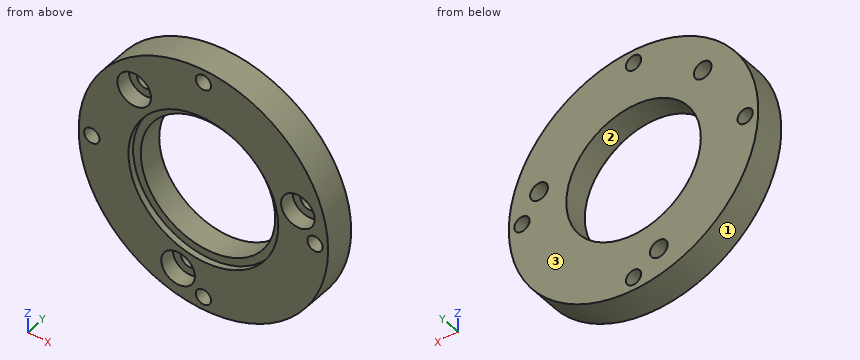
```python
from build123d import *

# Parameters (mm, degrees)
SKETCH_1_R                    = 20.4
SKETCH_1_R_2                  = 11
EXTRUDE_1_DEPTH               = 5
M3X0_51_D                     = 2.5
HOLE_WIZARD_M2_51_D           = 2.9
HOLE_WIZARD_M2_51_CBORE_D     = 5.5
HOLE_WIZARD_M2_51_CBORE_DEPTH = 2.5
SKETCH_9_R                    = 12.25
CUT_EXTRUDE_1_DEPTH           = 1


with BuildPart() as part:
    # Эскиз1 → Бобышка-Вытянуть1 (new body)
    with BuildSketch(Plane(origin=(0, 0, 0), x_dir=(1, 0, 0), z_dir=(0, 1, 0))):
        Circle(SKETCH_1_R)
        Circle(SKETCH_1_R_2, mode=Mode.SUBTRACT)
    extrude(amount=EXTRUDE_1_DEPTH)

    # Отверстие обработанное метчиком M3x0.51 (through all)
    with Locations(Plane(origin=(0, 5, 0), x_dir=(1, 0, 0), z_dir=(0, 1, 0))):
        with Locations((-18.25, 0), (0, 18.25), (18.25, 0), (0, -18.25)):
            Hole(M3X0_51_D / 2)

    # Цековка для винта с внутренним шестигранником M2.51 (through all)
    with Locations(Plane(origin=(0, 0, 0), x_dir=(-1, 0, 0), z_dir=(0, -1, 0))):
        with Locations((11.313708499, -11.313708499), (4.141104722, 15.454813221), (-15.454813221, -4.141104722)):
            CounterBoreHole(HOLE_WIZARD_M2_51_D / 2, HOLE_WIZARD_M2_51_CBORE_D / 2, HOLE_WIZARD_M2_51_CBORE_DEPTH)

    # Эскиз9 → Вырез-Вытянуть1 (cut)
    with BuildSketch(Plane.XZ):
        Circle(SKETCH_9_R)
    extrude(amount=-CUT_EXTRUDE_1_DEPTH, mode=Mode.SUBTRACT)


solid = part.part
```
Source: CAD feature listing. Evaluate the final solid. Frame: model axes, mm. Face numbers are marked on the shaded views. Round coordinates to 2 decimals unless told otherwise and drop trailing zeros. Order: outer loops, then holes, each group sorted by start corner. A loop starts at its lowest first (then second) coordinate and runs counter-clockwise, first axis right, second up. Notation, with made-up numbers: (1.25, 68) -> (49.25, 68) arc R23 ccw to (49.25, 79) -> close; hole circle Ø10 at (4.25, -9). An arc over 180 degrees is marked (long way). One line per item, written item: value. Start each with the question number.
Q1. Pin query (flat end, axial travel): pin 1 (4 mm diameter, centred on x = -18.25, z = 0, fed in from +Y); pin 2 (3.5 mm diameter, centred on x = 15.45, z = 4.14, fed in from -Y). Return the tip coordinate at first contact, or that it passes through.
Q2. Section query C-C (z = 18.25). Return the cut outline in (x, y), plus the area to 3 significant figures.
Q3. Draft query along Z for the marked faces 1, 2 and 3. Return one class per face: pulls with the +Z half, pulls with the -Z half, needs draft (parallel to the pull), parting line crosses it, or undercut.
Q4. Section query B-B (x = -18.25). Return the cut outline in (y, z), plus the area to 3 significant figures.
Q5. Section query D-D (x = 0). Return the cut outline in (y, z).
Q6. Material intervals for probe 1 along Z at (x, y) = (0, 1.1); probe 2 along X at (y, z) = (1.4, 9); probe 3 along X at (y, z) = (2, -17.5), sorted ascending.
Q7. Section query A-A (z = 5). Return the cut outline in (x, y), plus the area to 3 significant figures.
Findings below:
1. pin 1: y = 5
1. pin 2: y = 2.5
2. outline: (-9.12, 0) -> (-1.25, 0) -> (-1.25, 5) -> (-9.12, 5) -> close; (1.25, 0) -> (9.12, 0) -> (9.12, 5) -> (1.25, 5) -> close
2. area: 78.7 mm²
3. face 1: parting line crosses it
3. face 2: undercut
3. face 3: needs draft
4. outline: (0, -9.12) -> (5, -9.12) -> (5, -1.25) -> (0, -1.25) -> close; (0, 1.25) -> (5, 1.25) -> (5, 9.12) -> (0, 9.12) -> close
4. area: 78.7 mm²
5. outline: (0, -20.4) -> (5, -20.4) -> (5, -19.5) -> (0, -19.5) -> close; (0, -17) -> (5, -17) -> (5, -11) -> (1, -11) -> (1, -12.25) -> (0, -12.25) -> close; (0, 12.25) -> (1, 12.25) -> (1, 11) -> (5, 11) -> (5, 17) -> (0, 17) -> close; (0, 19.5) -> (5, 19.5) -> (5, 20.4) -> (0, 20.4) -> close
6. probe 1: -20.4 to -19.5, -17 to -11, 11 to 17, 19.5 to 20.4
6. probe 2: -18.31 to -12.8, -9.83 to -6.32, 6.32 to 18.31
6. probe 3: -10.48 to -5.98, -2.3 to -1, 1 to 10.48
7. outline: (-19.78, 0) -> (-11.18, 0) -> (-11.18, 1) -> (-9.8, 1) -> (-9.8, 5) -> (-19.78, 5) -> close; (9.8, 1) -> (11.18, 1) -> (11.18, 0) -> (12.84, 0) -> (12.84, 2.5) -> (14.29, 2.5) -> (14.29, 5) -> (9.8, 5) -> close; (16.62, 2.5) -> (18.07, 2.5) -> (18.07, 0) -> (19.78, 0) -> (19.78, 5) -> (16.62, 5) -> close
7. area: 78.1 mm²
